from build123d import *

# Parameters (mm, degrees)
EXTRUDE_1_DEPTH     = 60
SKETCH_2_R          = 18
EXTRUDE_2_DEPTH     = 40
SKETCH_3_R          = 11
EXTRUDE_3_DEPTH     = 2
SKETCH_4_R          = 4
EXTRUDE_4_DEPTH     = 17
SKETCH_5_R          = 1.5
CUT_EXTRUDE_1_DEPTH = 4
CUT_EXTRUDE_START   = -15
CUT_EXTRUDE_2_DEPTH = 15


with BuildPart() as part:
    # 草图1 → 凸台-拉伸1 (new body)
    with BuildSketch(Plane.XY):
        Polygon((-29.69848481, 0), (0, 29.69848481), (29.69848481, 0), (0, -29.69848481), align=None)
    extrude(amount=EXTRUDE_1_DEPTH)

    # 草图2 → 凸台-拉伸2 (add)
    with BuildSketch(Plane.XY.offset(60)):
        Circle(SKETCH_2_R)
    extrude(amount=EXTRUDE_2_DEPTH)

    # 草图3 → 凸台-拉伸3 (add)
    with BuildSketch(Plane.XY.offset(100)):
        Circle(SKETCH_3_R)
    extrude(amount=EXTRUDE_3_DEPTH)

    # 草图4 → 凸台-拉伸4 (add)
    with BuildSketch(Plane.XY.offset(102)):
        Circle(SKETCH_4_R)
    extrude(amount=EXTRUDE_4_DEPTH)

    # 草图5 → 切除-拉伸1 (cut)
    with BuildSketch(Plane.XY.offset(100)):
        with Locations((0, 14)):
            Circle(SKETCH_5_R)
        with Locations((14, 0)):
            Circle(SKETCH_5_R)
        with Locations((0, -14)):
            Circle(SKETCH_5_R)
        with Locations((-14, 0)):
            Circle(SKETCH_5_R)
    extrude(amount=-CUT_EXTRUDE_1_DEPTH, mode=Mode.SUBTRACT)

    # 草图6 → 切除-拉伸2 (cut)
    with BuildSketch(Plane.XY.offset(119).offset(CUT_EXTRUDE_START)):
        with BuildLine():
            Line((2.645751311, 3), (-2.645751311, 3))
            ThreePointArc((-2.645751311, 3), (0, 4), (2.645751311, 3))
        make_face()
    extrude(amount=CUT_EXTRUDE_2_DEPTH, mode=Mode.SUBTRACT)


solid = part.part
Verification items for the finished model (mm, model axes). A direction names the side the tool comes from. Give positions to 0.01 mm unless a question says otherwise; leave off trailing zeros. Loops run counter-clockwise (first coordinate to the right, second up) from the corner with the lowest first, then second, coordinate; pieces in that order, holes last.
1. Cross-section at D-D on z = 83. Record the cut outline in (x, y), and give its area (3 significant figures).
Derived:
outline: circle Ø36 at (0, 0)
area: 1,020 mm2
2. Release check for a two-part mould opening along Y. For faces 4 (the flat face through (-15.1, 14.6, 29.6)), 5 (the cylindrical face through (-0.325, 12.536, 98.028)), 6 (the cylindrical face through (-2.343, 17.847, 79.72)), 7 (the flat face through (0, 0, 119)) record: +Y half, -Y half, draft (parallel to the pull), parting line (faces both ways), or undercut.
Derived:
face 4: +Y half
face 5: undercut
face 6: parting line
face 7: draft
3. Cross-section at A-A on z = 20. Record the cut outline in (x, y).
Derived:
outline: (-29.7, 0) - (0, -29.7) - (29.7, 0) - (0, 29.7) - close
4. Cross-section at B-B on x = -7. Record the cut outline in (y, z).
Derived:
outline: (-22.7, 0) - (22.7, 0) - (22.7, 60) - (16.58, 60) - (16.58, 100) - (8.49, 100) - (8.49, 102) - (-8.49, 102) - (-8.49, 100) - (-16.58, 100) - (-16.58, 60) - (-22.7, 60) - close
5. Go/stop test with flat-tipped pins: P1, Ø5, axis at x = 21, z = 44, coming from the -Y side; P2, Ø6, axis at y = -23, z = 39.5, coming from the +X side; P3, Ø10, axis at x = -12.5, z = 78, coming from the -Y side; P4, Ø10, axis at x = -12.5, y = -3, coming from the -Z side. Record where each tip stops, or that it passes through.
Derived:
P1: stops at y = -11.2
P2: stops at x = 9.7
P3: stops at y = -16.36
P4: stops at z = 0
6. Tool access check on faces 1 (the flat face through (15.1, -14.6, 29.6)), 2 (the flat face through (-14, 0, 96)), 3 (the flat face through (0, 3, 111)). Record the directions out of +Z, -Z, +X, -X, +Y, -Y that give a thin tool (end or side, any length) a straight path to the whole face; none if there is none.
Derived:
face 1: +Z, -Z, +X, -Y
face 2: +Z
face 3: +Z, +X, -X, +Y
7. Cross-section at C-C on y = -14. Record the cut outline in (x, z).
Derived:
outline: (-15.7, 0) - (15.7, 0) - (15.7, 60) - (11.31, 60) - (11.31, 100) - (1.5, 100) - (1.5, 96) - (-1.5, 96) - (-1.5, 100) - (-11.31, 100) - (-11.31, 60) - (-15.7, 60) - close
8. Material ranges on probe 1 along Y at (x, z) = (0, 97.6); probe 2 along Z at (x, y) = (-8, 4); probe 3 along Z at (x, y) = (-22, 5.5), recorded low to high.
Derived:
probe 1: y = -18 to -15.5, -12.5 to 12.5, 15.5 to 18
probe 2: z = 0 to 102
probe 3: z = 0 to 60
